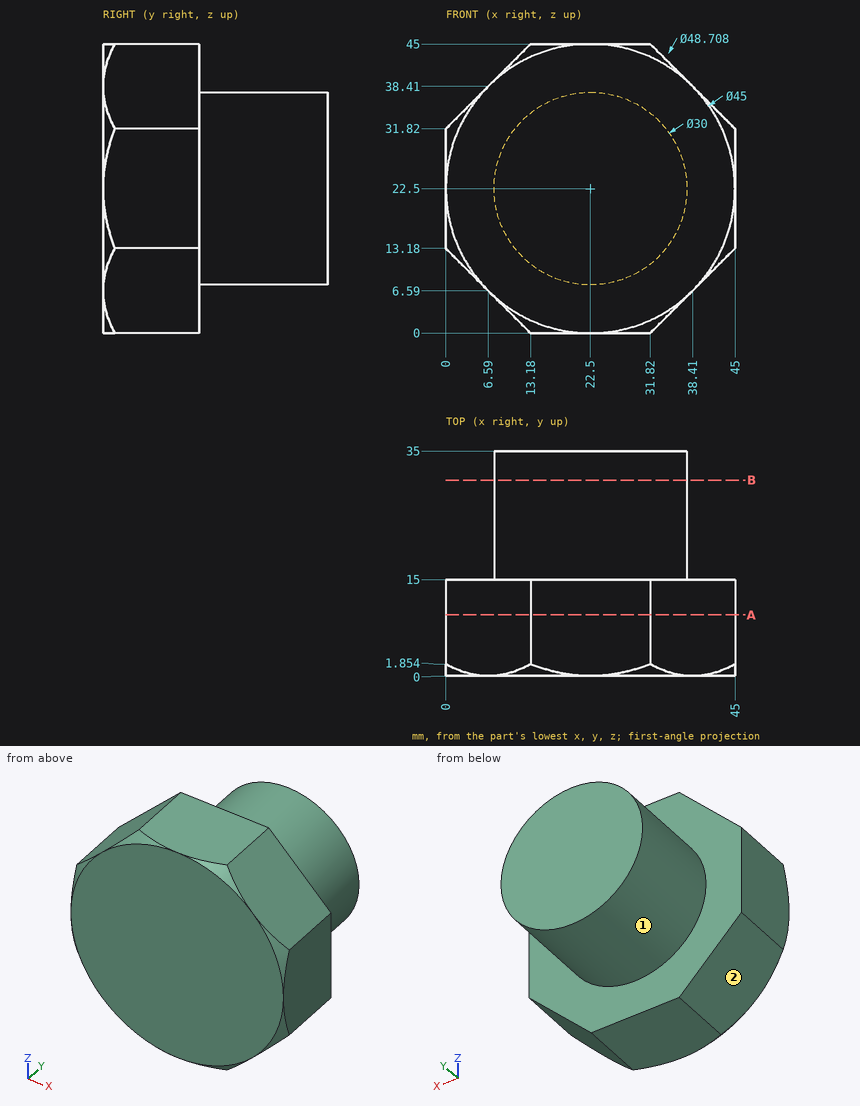
Part print with two shaded views. Sizes in mm from the minimum x, y, z corner. A direction names the side the tool comes from. Give positions to 0.01 mm unless a question says otherwise; leave off trailing zeros. Order: outer loops, then holes, each group sorted by start corner. A loop starts at its lowest first (then second) coordinate and runs counter-clockwise, first axis right, second up.
(1) Saw through at A-A, the plane y = 9.5. Give the cut face in (x, z).
(2) Tool access for the marked faces 1 and 2: list every direction of +Z, -Z, +X, -X, +Y, -Y with a clear straight run to the whole face (end or side of a thin tool).
(3) Flat gauge pins, fed straight in: pin 1 (6 mm diameter, centred on x = 36.5, y = 4, fed in from +Z); pin 2 (10 mm diameter, centred on y = 30, z = 14, fed in from -X); pin 3 (12 mm diameter, centred on y = 28, z = 15.5, fed in from -X). Where does each tip first touch, or does it go through?
(4) Drill centre lines: L1, parallel to Y at x = 32.5, z = 8.5; L2, parallel to X at y = 19, z = 22.5; L3, parallel to X at y = 24.5, z = 15. Where is each one in solid material? Low to high.
(5) Saw through at B-B, the plane y = 30.5. Give the cut face in (x, z), then the cut area to 3 significant figures.
Results found:
1. outline: (0, 13.18) - (13.18, 0) - (31.82, 0) - (45, 13.18) - (45, 31.82) - (31.82, 45) - (13.18, 45) - (0, 31.82) - close
2. face 1: +Y
2. face 2: -Z, -X, +Y, -Y
3. pin 1: stops at z = 43.32
3. pin 2: stops at x = 7.91
3. pin 3: stops at x = 7.53
4. L1: y = 0 to 15
4. L2: x = 7.5 to 37.5
4. L3: x = 9.51 to 35.49
5. outline: circle Ø30 at (22.5, 22.5)
5. area: 707 mm2
